Here's how the part is built. I have some questions about the finished solid (model axes, mm). Give positions to 0.01 mm unless a question says otherwise; leave off trailing zeros. Loops run counter-clockwise (first coordinate to the right, second up) from the corner with the lowest first, then second, coordinate; pieces in that order, holes last. Notation, with made-up numbers: (45.25, 23) - (85.25, 23) arc R14 ccw to (85.25, 32) - close; hole circle Ø9 at (69.25, 3.5). An arc over 180 degrees is marked (long way). Use a Markdown table: item, result.
from build123d import *

# Parameters (mm, degrees)
F0_R     = 10.445
F0_R_2   = 9.445
F1_DEPTH = 6
F2_SIZE  = 0.508
F3_SIZE  = 0.254


with BuildPart() as f1:
    # F0 (on Top) → F1 (new body)
    with BuildSketch(Plane.XY):
        Circle(F0_R)
        Circle(F0_R_2, mode=Mode.SUBTRACT)
    extrude(amount=F1_DEPTH)

    # F2
    f2_edges = [f1.edges().sort_by_distance(p)[0] for p in [
        (-9.445, 0, 6),
        (-9.445, 0, 0),
    ]]
    chamfer(f2_edges, length=F2_SIZE)

    # F3
    f3_edges = [f1.edges().sort_by_distance(p)[0] for p in [
        (-10.445, 0, 6),
        (-10.445, 0, 0),
    ]]
    chamfer(f3_edges, length=F3_SIZE)


solid = f1.part
(1) We'd pull the mould along X, two halves only. Please class faces 1 (the face through (-1.23, 9.365, 2.965)), 2 (the face through (-8.289, -6.356, 2.962)): pulls with the +X half, pulls with the -X half, needs draft (parallel to the pull), parting line crosses it, or undercut.
A:
| item | result |
|---|---|
| face 1 | undercut |
| face 2 | parting line crosses it |
(2) If I drill on line 1 (Y direction, x = 0, z = 1.9) (3 decimals); line 2 (Y direction, x = 8.5, z = 2.35); line 3 (X direction, y = 6.5, z = 3), over which ranges is the centre line in solid material (lowest first)?
A:
| item | result |
|---|---|
| line 1 | -10.445 to -9.445, 9.445 to 10.445 |
| line 2 | -6.07 to -4.12, 4.12 to 6.07 |
| line 3 | -8.18 to -6.85, 6.85 to 8.18 |
(3) Suppose I cut it at C-C on z = 5. Write out the boundary of the cut face in (x, y) (3 decimals), plus the area to 3 significant figures.
A:
| item | result |
|---|---|
| outline | circle Ø20.89 at (0, 0); hole circle Ø18.89 at (0, 0) |
| area | 62.5 mm2 |
(4) Will these pins go through, and if not, where does the flat tip stop? pin 1 (1.5 mm diameter, centred on y = 2, z = 3.5, fed in from +X); pin 2 (3 mm diameter, centred on x = 4, y = -6.5, fed in from +Z); pin 3 (12 mm diameter, centred on x = 7, y = 6.5, fed in from -Z); pin 4 (3 mm diameter, centred on y = 4, z = 4, fed in from -X).
A:
| item | result |
|---|---|
| pin 1 | x = 10.37 |
| pin 2 | through |
| pin 3 | z = 0 |
| pin 4 | x = -10.14 |
(5) Suppose I cut it at A-A on x = 0. Write out the boundary of the cut face in (y, z) (3 decimals), plus the area to 3 significant figures.
A:
| item | result |
|---|---|
| outline | (-10.445, 0.254) - (-10.191, 0) - (-9.953, 0) - (-9.445, 0.508) - (-9.445, 5.492) - (-9.953, 6) - (-10.191, 6) - (-10.445, 5.746) - close; (9.445, 0.508) - (9.953, 0) - (10.191, 0) - (10.445, 0.254) - (10.445, 5.746) - (10.191, 6) - (9.953, 6) - (9.445, 5.492) - close |
| area | 11.4 mm2 |
